Could you check a few things on this model? Use its own coordinates, in mm. Face numbers are marked on the shaded views. A direction names the side the tool comes from. Round coordinates to 2 decimals unless told otherwise and drop trailing zeros. Loops run counter-clockwise (first coordinate to the right, second up) from the corner with the lowest first, then second, coordinate; pieces in that order, holes last. Notation, with made-up numbers: M 44.5,34 L 49.5,34 A35 ccw 49.5,67 Z; hole C -32,44 d5. An arc over 180 degrees is marked long. Return JSON: item names as keys, results as strings. Group by question number.
```python
from build123d import *

# Parameters (mm, degrees)
F1_DEPTH = 6.35
F2_W     = 1.395
F2_H     = 0.71
F3_DEPTH = 0.3
F4_W     = 0.81
F4_H     = 1.57
F5_DEPTH = 0.3


with BuildPart() as f1:
    # F0 (on Right) → F1 (new body)
    with BuildSketch(Plane.YZ):
        with BuildLine():
            Line((-7.34, 0), (0, 0))
            Line((0, 0), (0, 0.3))
            Line((0, 0.3), (-7.04, 0.3))
            Line((-7.04, 0.3), (-7.04, 13.800869))
            ThreePointArc((-7.04, 13.800869), (-7.703292, 14.653092), (-8.692279, 14.219335))
            Line((-8.692279, 14.219335), (-11, 9.955639))
            Line((-11, 9.955639), (-10.607156, 7.06))
            Line((-10.607156, 7.06), (-10.309879, 7.100331))
            Line((-10.309879, 7.100331), (-10.68956, 9.898947))
            Line((-10.68956, 9.898947), (-8.428445, 14.076535))
            ThreePointArc((-8.428445, 14.076535), (-7.776946, 14.362275), (-7.34, 13.800869))
            Line((-7.34, 13.800869), (-7.34, 0))
        make_face()
    extrude(amount=F1_DEPTH)

    # F2 (on face) → F3 (cut, through all)
    with BuildSketch(Plane.XZ.offset(7.34)):
        with Locations((5.6525, 0.655)):
            Rectangle(F2_W, F2_H)
        with Locations((0.6975, 0.655)):
            Rectangle(F2_W, F2_H)
    extrude(amount=-F3_DEPTH, mode=Mode.SUBTRACT)

    # F4 (on face) → F5 (cut, through all)
    with BuildSketch(Plane.XY.offset(0.3)):
        Polygon((0, -4.32), (0, -7.34), (1.395, -7.34), (1.395, -7.04), (1.395, -4.32), align=None)
        Polygon((4.955, -4.32), (4.955, -7.04), (4.955, -7.34), (6.35, -7.34), (6.35, -4.32), align=None)
        with Locations((3.175, -2.263539)):
            Rectangle(F4_W, F4_H)
    extrude(amount=-F5_DEPTH, mode=Mode.SUBTRACT)


solid = f1.part
```
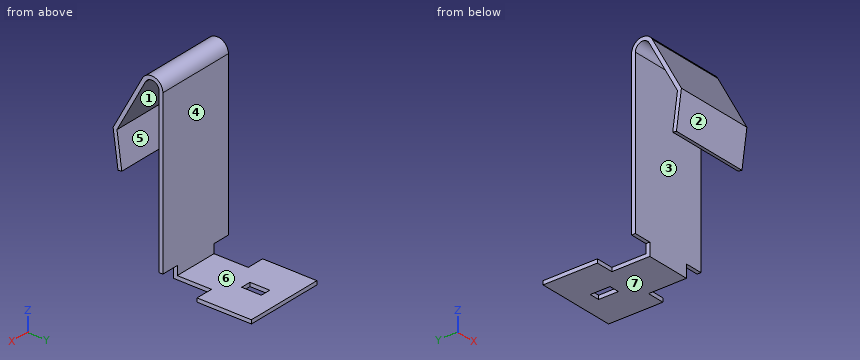
1. I need wall thicknesses on probe 1 along Z at (x, y) = (2, -6.5); probe 2 along Y at (x, z) = (1.75, 2.25); probe 3 along Y at (x, z) = (1.25, 7.5). Which ranges of each line are inside material? Lowest first, please.
2. If we section it at B-B, the plane x = 3.25: Please give me the cut outline in (y, z).
3. If we section it at C-C, the plane x = 2: Please give me the cut outline in (y, z), then the cut area to 3 significant figures.
4. We'd pull the mould along Y, two halves only. Please class the marked faces 1, 2, 3 and 4: +Y half, -Y half, draft (parallel to the pull), parting line (faces both ways), or undercut.
5. If we section it at D-D, the plane x = 1: Please give me the cut outline in (y, z).
6. If we section it at A-A, the plane y = -2.5: Please give me the cut outline in (x, z).
7. I'm going to push flat-ended pins straight in: pin 1 Ø0.8 at (y, z) = (-6, 0.5) entering from -X (3 decimals); pin 2 Ø0.5 at (y, z) = (-5, 0.5) entering from +X (3 decimals); pin 3 Ø1.5 at (x, y) = (2.5, -9) entering from +Z. Where does each tip first touch, or does it pass through?
8. On a 3-axis mill with a long thin cutter (end or side, diameter ignored), from which of +Z, -Z, +X, -X, +Y, -Y can I reach the whole of each face in a straight line? I mean the marked faces 5, 6 and 7. Say none if no direction works.
Geometry results:
{
 "1": {"probe 1": "0 to 0.3", "probe 2": "-7.34 to -7.04", "probe 3": "-10.67 to -10.36, -7.34 to -7.04"},
 "2": {"outline": "M -11,9.96 L -10.61,7.06 L -10.31,7.1 L -10.69,9.9 L -8.43,14.08 A0.58 cw -7.34,13.8 L -7.34,0 L -3.05,0 L -3.05,0.3 L -7.04,0.3 L -7.04,13.8 A0.88 ccw -8.69,14.22 Z; M -1.48,0 L 0,0 L 0,0.3 L -1.48,0.3 Z"},
 "3": {"outline": "M -11,9.96 L -10.61,7.06 L -10.31,7.1 L -10.69,9.9 L -8.43,14.08 A0.58 cw -7.34,13.8 L -7.34,0 L 0,0 L 0,0.3 L -7.04,0.3 L -7.04,13.8 A0.88 ccw -8.69,14.22 Z", "area": "9.13 mm^2"},
 "4": {"face 1": "undercut", "face 2": "-Y half", "face 3": "undercut", "face 4": "+Y half"},
 "5": {"outline": "M -11,9.96 L -10.61,7.06 L -10.31,7.1 L -10.69,9.9 L -8.43,14.08 A0.58 cw -7.34,13.8 L -7.34,1.01 L -7.04,1.01 L -7.04,13.8 A0.88 ccw -8.69,14.22 Z; M -4.32,0 L 0,0 L 0,0.3 L -4.32,0.3 Z"},
 "6": {"outline": "M 0,0 L 2.77,0 L 2.77,0.3 L 0,0.3 Z; M 3.58,0 L 6.35,0 L 6.35,0.3 L 3.58,0.3 Z"},
 "7": {"pin 1": "x = 1.395", "pin 2": "x = 4.955", "pin 3": "z = 14.62"},
 "8": {"face 5": "+X, -X", "face 6": "+Z, +X, -X, +Y", "face 7": "-Z, +X, -X, +Y, -Y"}
}
